```python
from build123d import *

# Parameters (mm, degrees)
SKETCH1_R           = 7
BOSS_EXTRUDE1_DEPTH = 5


with BuildPart() as part:
    # Sketch1 → Boss-Extrude1 (new body)
    with BuildSketch(Plane.XY):
        with BuildLine():
            Line((1502.640695659, 642.154083815), (1502.640695659, 267.552169785))
            Line((1502.640695659, 267.552169785), (-27.359304341, 267.552169785))
            Line((-27.359304341, 267.552169785), (-27.359304341, 2512.552169785))
            Line((-27.359304341, 2512.552169785), (201.640695659, 2512.552169785))
            ThreePointArc((201.640695659, 2512.552169785), (558.874686731, 1373.364959534), (1502.640695659, 642.154083815))
        make_face()
        with Locations((1446.640695659, 292.552169785)):
            Circle(SKETCH1_R, mode=Mode.SUBTRACT)
        with Locations((1146.640695659, 292.552169785)):
            Circle(SKETCH1_R, mode=Mode.SUBTRACT)
        with Locations((846.640695659, 292.552169785)):
            Circle(SKETCH1_R, mode=Mode.SUBTRACT)
        with Locations((546.640695659, 292.552169785)):
            Circle(SKETCH1_R, mode=Mode.SUBTRACT)
        with Locations((246.640695659, 292.552169785)):
            Circle(SKETCH1_R, mode=Mode.SUBTRACT)
        with Locations((46.640695659, 292.552169785)):
            Circle(SKETCH1_R, mode=Mode.SUBTRACT)
        with Locations((-2.359304341, 362.552169785)):
            Circle(SKETCH1_R, mode=Mode.SUBTRACT)
        with Locations((-2.359304341, 562.552169785)):
            Circle(SKETCH1_R, mode=Mode.SUBTRACT)
        with Locations((-2.359304341, 862.552169785)):
            Circle(SKETCH1_R, mode=Mode.SUBTRACT)
        with Locations((-2.359304341, 1162.552169785)):
            Circle(SKETCH1_R, mode=Mode.SUBTRACT)
        with Locations((-2.359304341, 1462.552169785)):
            Circle(SKETCH1_R, mode=Mode.SUBTRACT)
        with Locations((-2.359304341, 1762.552169785)):
            Circle(SKETCH1_R, mode=Mode.SUBTRACT)
        with Locations((-2.359304341, 2062.552169785)):
            Circle(SKETCH1_R, mode=Mode.SUBTRACT)
        with Locations((-2.359304341, 2362.552169785)):
            Circle(SKETCH1_R, mode=Mode.SUBTRACT)
        with Locations((572.640695659, 717.552169785)):
            Circle(SKETCH1_R, mode=Mode.SUBTRACT)
        with Locations((637.640695659, 717.552169785)):
            Circle(SKETCH1_R, mode=Mode.SUBTRACT)
        with Locations((572.640695659, 797.552169785)):
            Circle(SKETCH1_R, mode=Mode.SUBTRACT)
        with Locations((637.640695659, 797.552169785)):
            Circle(SKETCH1_R, mode=Mode.SUBTRACT)
        with BuildLine():
            Line((190.238398333, 2349.629423417), (189.453807376, 2359.598596754))
            ThreePointArc((189.453807376, 2359.598596754), (181.926172369, 2366.02780442), (175.496964703, 2358.500169414))
            Line((175.496964703, 2358.500169414), (176.281555661, 2348.530996076))
            ThreePointArc((176.281555661, 2348.530996076), (183.809190667, 2342.10178841), (190.238398333, 2349.629423417))
        make_face(mode=Mode.SUBTRACT)
        with BuildLine():
            Line((240.427272718, 2037.764802741), (238.092819079, 2047.488501945))
            ThreePointArc((238.092819079, 2047.488501945), (229.652112089, 2052.660973841), (224.479640194, 2044.220266851))
            Line((224.479640194, 2044.220266851), (226.814093832, 2034.496567648))
            ThreePointArc((226.814093832, 2034.496567648), (235.254800822, 2029.324095752), (240.427272718, 2037.764802741))
        make_face(mode=Mode.SUBTRACT)
        with BuildLine():
            Line((338.784613876, 1737.591022772), (334.957779552, 1746.829818097))
            ThreePointArc((334.957779552, 1746.829818097), (325.811838798, 1750.618190798), (322.023466097, 1741.472250044))
            Line((322.023466097, 1741.472250044), (325.85030042, 1732.233454719))
            ThreePointArc((325.85030042, 1732.233454719), (334.996241175, 1728.445082018), (338.784613876, 1737.591022772))
        make_face(mode=Mode.SUBTRACT)
        with BuildLine():
            Line((482.888537638, 1456.49935819), (477.663551991, 1465.025759834))
            ThreePointArc((477.663551991, 1465.025759834), (468.037581727, 1467.33674966), (465.72658969, 1457.710779928))
            Line((465.72658969, 1457.710779928), (470.951575337, 1449.184378284))
            ThreePointArc((470.951575337, 1449.184378284), (480.57754644, 1446.873387087), (482.888537638, 1456.49935819))
        make_face(mode=Mode.SUBTRACT)
        with BuildLine():
            Line((669.190727148, 1201.411218669), (662.696246664, 1209.015278325))
            ThreePointArc((662.696246664, 1209.015278325), (652.827268567, 1209.791983746), (652.050563146, 1199.923005648))
            Line((652.050563146, 1199.923005648), (658.545043629, 1192.318945992))
            ThreePointArc((658.545043629, 1192.318945992), (668.414021727, 1191.542240571), (669.190727148, 1201.411218669))
        make_face(mode=Mode.SUBTRACT)
        with BuildLine():
            Line((893.103804198, 978.607720791), (885.499744542, 985.102201274))
            ThreePointArc((885.499744542, 985.102201274), (875.630766445, 984.325495853), (876.407471866, 974.456517756))
            Line((876.407471866, 974.456517756), (884.011531522, 967.962037273))
            ThreePointArc((884.011531522, 967.962037273), (893.880509619, 968.738742693), (893.103804198, 978.607720791))
        make_face(mode=Mode.SUBTRACT)
        with BuildLine():
            Line((1149.114285708, 793.575026117), (1140.587884064, 798.800011764))
            ThreePointArc((1140.587884064, 798.800011764), (1130.961912961, 796.489020567), (1133.272904158, 786.863049463))
            Line((1133.272904158, 786.863049463), (1141.799305802, 781.638063816))
            ThreePointArc((1141.799305802, 781.638063816), (1151.425276905, 783.949055014), (1149.114285708, 793.575026117))
        make_face(mode=Mode.SUBTRACT)
        with BuildLine():
            Line((1430.918343971, 650.869253678), (1421.679548646, 654.696088002))
            ThreePointArc((1421.679548646, 654.696088002), (1412.533607891, 650.907715301), (1416.321980592, 641.761774547))
            Line((1416.321980592, 641.761774547), (1425.560775918, 637.934940223))
            ThreePointArc((1425.560775918, 637.934940223), (1434.706716672, 641.723312924), (1430.918343971, 650.869253678))
        make_face(mode=Mode.SUBTRACT)
    extrude(amount=BOSS_EXTRUDE1_DEPTH)


solid = part.part
```
Part model, mm, in its own coordinate system. Coordinates: 2 decimals unless noted, no trailing zeros. Write each loop counter-clockwise with the first axis right and the second up, starting at its lowest first coordinate (ties: lowest second). Pieces come first, ordered by that corner, then holes.
Item 1: Slice it at B-B (x = 980). Write the cut outline in (y, z).
Item 2: Slice it at C-C (y = 2095). Write the cut outline in (x, z).
Item 3: Probe line 1 (X direction, y = 788, z = 2.75); line 2 (X direction, y = 1101.5, z = 3.7); line 3 (Y direction, x = 357, z = 4.1). List the from-to ranges inside material, lowest first.
Item 4: Slice it at A-A (z = 3.4). Count the separate pieces of the cut face and the enclosed holes in it, and give its area (3 significant figures).
Item 5: Pin check, flat tip, straight feed: pin 1 (12.5 mm diameter, centred on x = -2.36, y = 1162.55, fed in from -Z). Stop position of the tip, or through.
Results found:
1. outline: (267.55, 0) - (931.47, 0) - (931.47, 5) - (267.55, 5) - close
2. outline: (-27.36, 0) - (245.83, 0) - (245.83, 5) - (-27.36, 5) - close
3. line 1: x = -27.36 to 1131.87, 1152.45 to 1193.67
3. line 2: x = -27.36 to 786.34
3. line 3: y = 267.55 to 1740.71
4. separate pieces: 1
4. enclosed holes: 26
4. area: 1,660,000 mm2
5. pin 1: passes through
